from build123d import *

# Parameters (mm, degrees)
SKETCH_R     = 16.8
PAD_DEPTH    = 24
SKETCH001_R  = 15.19
PAD001_DEPTH = 30
SKETCH002_R  = 1
PAD002_DEPTH = 12


with BuildPart() as part:
    # Sketch → Pad (new body)
    with BuildSketch(Plane.XY):
        Circle(SKETCH_R)
    extrude(amount=PAD_DEPTH)

    # Sketch001 → Pad001 (new body)
    with BuildSketch(Plane.XY.offset(24)):
        Circle(SKETCH001_R)
    extrude(amount=PAD001_DEPTH)

    # Sketch002 → Pad002 (new body)
    with BuildSketch(Plane.XY.offset(54)):
        with Locations((-9.2, 0)):
            Circle(SKETCH002_R)
    extrude(amount=PAD002_DEPTH)


solid = part.part
Here's how the part is built. I have some questions about the finished solid (model axes, mm). A direction names the side the tool comes from. Round coordinates to 2 decimals unless told otherwise and drop trailing zeros. Loops run counter-clockwise (first coordinate to the right, second up) from the corner with the lowest first, then second, coordinate; pieces in that order, holes last. Notation, with made-up numbers: (3, 38.25) - (49, 38.25) arc R15 cw to (49, 44.25) - close; hole circle Ø3 at (29.25, 55.25). An arc over 180 degrees is marked (long way). One line per question, with ' | ' between items. Start each with the question number.
Q1. Please list where these lines run through material, in increasing order: line 1 (Z direction, x = 9.5, y = -7.5); line 2 (Y direction, x = -8, z = 9.5); line 3 (X direction, y = -8.5, z = 47). Write a range as [from, to].
Q2. I want a section at D-D (y = -10). Write out the boundary of the cut face in (x, z), then the cut area to 3 significant figures.
Q3. I want a section at A-A (x = 0). Write out the boundary of the cut face in (y, z), then the cut area to 3 significant figures.
Q4. For faces 1 (the flat face through (-9, 0, 66)), 2 (the cylindrical face through (-11.196, 10.266, 38.79)), which set-ups out of +Z, -Z, +X, -X, +Y, -Y let a thin tool reach every point of the face, with its end or its side?
Q5. I want a section at B-B (y = 0). Write out the boundary of the cut face in (x, z), then the cut area to 3 significant figures.
Q6. I want a section at C-C (z = 34.5). Write out the boundary of the cut face in (x, y), then the cut area to 3 significant figures.
Q7. Will these pins go through, and if not, where does the flat tip stop? pin 1 (3 mm diameter, centred on y = -10.5, z = 36.5, fed in from +X); pin 2 (1.5 mm diameter, centred on x = 10.5, y = -2.5, fed in from +Z); pin 3 (5 mm diameter, centred on x = 13.5, z = 23, fed in from +Y); pin 4 (4 mm diameter, centred on y = -4.5, z = 57.5, fed in from -X).
Response values:
1) line 1: z = [0, 54] | line 2: y = [-14.77, 14.77] | line 3: x = [-12.59, 12.59]
2) outline: (-13.5, 0) - (13.5, 0) - (13.5, 24) - (11.43, 24) - (11.43, 54) - (-11.43, 54) - (-11.43, 24) - (-13.5, 24) - close | area: 1,330 mm²
3) outline: (-16.8, 0) - (16.8, 0) - (16.8, 24) - (15.19, 24) - (15.19, 54) - (-15.19, 54) - (-15.19, 24) - (-16.8, 24) - close | area: 1,720 mm²
4) face 1: +Z, +X, -X, +Y, -Y | face 2: +Z
5) outline: (-16.8, 0) - (16.8, 0) - (16.8, 24) - (15.19, 24) - (15.19, 54) - (-8.2, 54) - (-8.2, 66) - (-10.2, 66) - (-10.2, 54) - (-15.19, 54) - (-15.19, 24) - (-16.8, 24) - close | area: 1,740 mm²
6) outline: circle Ø30.38 at (0, 0) | area: 725 mm²
7) pin 1: stops at x = 12.24 | pin 2: stops at z = 54 | pin 3: stops at y = 12.7 | pin 4: passes through
